Could you check a few things on this model? Use its own coordinates, in mm. Face numbers are marked on the shaded views. Give positions to 0.01 mm unless a question says otherwise; leave off trailing zeros. Loops run counter-clockwise (first coordinate to the right, second up) from the corner with the lowest first, then second, coordinate; pieces in that order, holes last. Notation, with made-up numbers: (88.25, 22.25) - (103.25, 22.25) arc R16 cw to (103.25, 46.25) - close; hole circle Ø9 at (69.5, 12.5). An arc over 180 degrees is marked (long way). Write each question's results on one line, items separated by ' | '. Start each with the question number.
(1) Suppose I cut it at A-A (z = 9). Please give me the cut outline in (x, y), and give its area (3 significant figures).
(2) For pin 1 (0.7 mm diameter, centred on y = 2, z = -7.5, fed in from +X); pin 2 (0.5 mm diameter, centred on y = 2, z = 6.5, fed in from -X); pin 3 (1 mm diameter, centred on x = -15.5, y = 1.5, fed in from +Z), each with a flat end and sliding along its axis, tell me the tip position at first contact or that it passes through.
(3) Suppose I cut it at B-B (x = 9). Please give me the cut outline in (y, z).
(4) Suppose I cut it at C-C (y = 1.2). Please give me the cut outline in (x, z).
(5) Suppose I cut it at D-D (z = -4.5). Please give me the cut outline in (x, y).
(6) If we mould it in two halves opening along X, with no side actions, what happens to the marked faces 1, 2 and 3? For each: released by +X, released by -X, zero draft, split by the parting line, or undercut.
(7) I need wall thicknesses on line 1 (Z direction, x = -1, y = 2.2); line 2 (X direction, y = 1.4, z = -0.5); line 3 (Y direction, x = -7, z = 2). Which ranges of each line are inside material? Lowest first, please.
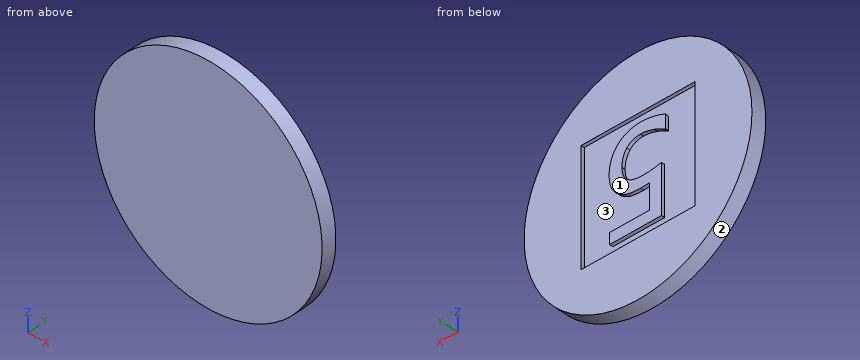
Autodesk Inventor part; units mm, degrees
ref_plane "YZ Plane" through (0, 0, 0) normal (1, 0, 0) x (0, 1, 0)
ref_plane "XZ Plane" through (0, 0, 0) normal (0, 1, 0) x (-1, 0, 0)
ref_plane "XY Plane" through (0, 0, 0) normal (0, 0, 1) x (1, 0, 0)
sketch "Sketch1" plane through (0, 0, 0) normal (0, 1, 0) x (-1, 0, 0)
  circle A0 centre (0, 0) radius 20
  dimension "d0" = 40
extrude "Extrusion1" add sketch "Sketch1" along normal blind 2.6
sketch "Sketch2" plane through (0, 2.6, 0) normal (0, 1, 0) x (1, 0, 0)
  line L0 (10, -10) -> (-10, -10)
  line L1 (-10, -10) -> (-10, 10)
  line L2 (-10, 10) -> (10, 10)
  line L3 (10, 10) -> (10, -10)
  line L4 (10, -10) -> (-10, 10) construction
  line L5 (-10, -10) -> (10, 10) construction
  point P0 (0, 0)
  dimension "d3" = 20
  dimension "d4" = 20
extrude "Extrusion2" cut sketch "Sketch2" against normal blind 0.6
sketch "Sketch4" plane through (0, 2, 0) normal (0, 1, 0) x (1, 0, 0)
  line L0 (-6.192, 8.5476) -> (6.2647, 8.5476) construction
  line L1 (6.2647, 8.5476) -> (6.2647, -8.4022) construction
  line L2 (6.2647, -8.4022) -> (-6.192, -8.4022) construction
  line L3 (-6.192, -8.4022) -> (-6.192, 8.5476) construction
  spline S0 degree 2 poles (5.0809, -2.7792) (5.0809, -3.9764) (4.3141, -6.0211) (3.6146, -6.7745) knots 0 0 0 1 2 2 2
  spline S1 degree 2 poles (3.6146, -6.7745) (2.9151, -7.5278) (0.83, -8.4022) (-0.4614, -8.4022) knots 0 0 0 1 2 2 2
  spline S2 degree 2 poles (-0.4614, -8.4022) (-1.6452, -8.4022) (-3.9589, -7.8775) (-4.8064, -7.4605) knots 0 0 0 1 2 2 2
  line L4 (-4.8064, -7.4605) -> (-4.8064, -5.1064)
  line L5 (-4.8064, -5.1064) -> (-4.645, -5.1064)
  spline S3 degree 2 poles (-4.645, -5.1064) (-4.3894, -5.2947) (-3.4343, -5.779) (-2.8559, -5.9942) knots 0 0 0 1 2 2 2
  spline S4 degree 2 poles (-2.8559, -5.9942) (-2.1967, -6.2229) (-1.1071, -6.4785) (-0.421, -6.4785) knots 0 0 0 1 2 2 2
  spline S5 degree 2 poles (-0.421, -6.4785) (0.2516, -6.4785) (1.5161, -5.9942) (1.9735, -5.4696) knots 0 0 0 1 2 2 2
  spline S6 degree 2 poles (1.9735, -5.4696) (2.3905, -4.9719) (2.821, -3.6536) (2.821, -2.7657) knots 0 0 0 1 2 2 2
  spline S7 degree 2 poles (2.821, -2.7657) (2.821, -1.8779) (2.3367, -0.7479) (1.8793, -0.3712) knots 0 0 0 1 2 2 2
  spline S8 degree 2 poles (1.8793, -0.3712) (1.4085, 0.0458) (0.0094, 0.3956) (-0.838, 0.3956) knots 0 0 0 1 2 2 2
  spline S9 degree 2 poles (-0.838, 0.3956) (-1.7528, 0.3956) (-3.5688, 0.1131) (-4.1204, -0.008) knots 0 0 0 1 2 2 2
  line L6 (-4.1204, -0.008) -> (-4.1204, 8.5476)
  line L7 (-4.1204, 8.5476) -> (4.9868, 8.5476)
  line L8 (4.9868, 8.5476) -> (4.9868, 6.597)
  line L9 (4.9868, 6.597) -> (-1.9815, 6.597)
  line L10 (-1.9815, 6.597) -> (-1.9815, 2.1712)
  spline S10 degree 2 poles (-1.9815, 2.1712) (-1.5779, 2.2251) (-0.7977, 2.2654) (-0.4748, 2.2654) knots 0 0 0 1 2 2 2
  spline S11 degree 2 poles (-0.4748, 2.2654) (0.8031, 2.2654) (2.5654, 1.8484) (3.3725, 1.2296) knots 0 0 0 1 2 2 2
  spline S12 degree 2 poles (3.3725, 1.2296) (4.1931, 0.6108) (5.0809, -1.2725) (5.0809, -2.7792) knots 0 0 0 1 2 2 2
extrude "Extrusion4" add sketch "Sketch4" along normal blind 0.6
properties part number "TopMarker1"
Output values:
1) outline: (-17.86, 0) - (17.86, 0) - (17.86, 2.6) - (10, 2.6) - (10, 2) - (-10, 2) - (-10, 2.6) - (-17.86, 2.6) - close | area: 80.9 mm2
2) pin 1: x = 18.68 | pin 2: x = -19 | pin 3: z = 13.23
3) outline: (0, -17.86) - (2.6, -17.86) - (2.6, -10) - (2, -10) - (2, 10) - (2.6, 10) - (2.6, 17.86) - (0, 17.86) - close
4) outline: circle Ø40 at (0, 0)
5) outline: (-19.49, 0) - (19.49, 0) - (19.49, 2.6) - (10, 2.6) - (10, 2) - (-1.98, 2) - (-1.98, 2.6) - (-4.12, 2.6) - (-4.12, 2) - (-10, 2) - (-10, 2.6) - (-19.49, 2.6) - close
6) face 1: zero draft | face 2: split by the parting line | face 3: undercut
7) line 1: -19.97 to -10, -8.55 to -6.6, -2.25 to -0.39, 6.45 to 8.39, 10 to 19.97 | line 2: -19.99 to 19.99 | line 3: 0 to 2
